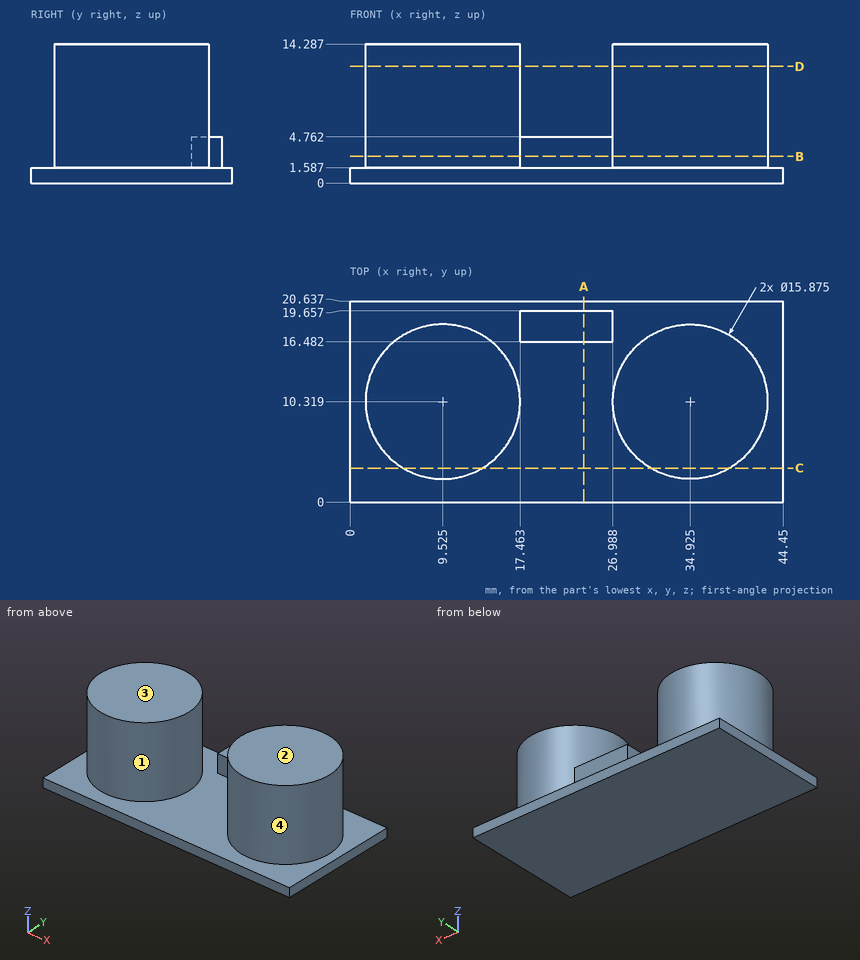
Could you check a few things on this drawing? It's one solid part, dimensions in mm from its lowest x, y, z. A direction names the side the tool comes from. Give positions to 0.01 mm unless a question says otherwise; leave off trailing zeros. Order: outer loops, then holes, each group sorted by start corner. A loop starts at its lowest first (then second) coordinate and runs counter-clockwise, first axis right, second up. Notation, with made-up numbers: (-12.75, 47) - (39.25, 47) arc R21 cw to (39.25, 71) - close; hole circle Ø8 at (6, 11). An arc over 180 degrees is marked (long way). Return JSON: item names as keys, results as strings. Group by question number.
Q1. Will these pins go through, and if not, where does the flat tip stop? pin 1 Ø3 at (y, z) = (18.5, 5) entering from -X; pin 2 Ø2.5 at (x, y) = (20, 17.5) entering from +Z; pin 3 Ø4 at (x, z) = (10.5, 6.5) entering from +Y.
Q2. Suppose I cut it at A-A, the plane x = 24. Please give me the cut outline in (y, z).
Q3. Which directions (+Z, -Z, +X, -X, +Y, -Y) give clear straight access to the entire face, cutting with the end or side of a thin tool? Please do the marked faces 1 and 2.
Q4. Suppose I cut it at B-B, the plane z = 2.75. Please give me the cut outline in (x, y) (1 decimal), and give its area (3 significant figures).
Q5. Please list where these lines run through material, in increasing order: line 1 along Z through (x, y) = (19.5, 1.5); line 2 along X through (y, z) = (6, 3.25) (1 decimal); line 3 along X through (y, z) = (5, 7.25) (1 decimal). Write a range as [from, to].
Q6. Thinking about a two-plate mould opening in X: for the marked faces 3 and 4, which applies, pulls with the +X half, pulls with the -X half, needs draft (parallel to the pull), parting line crosses it, or undercut?
Q7. Suppose I cut it at C-C, the plane y = 3.5. Please give me the cut outline in (x, z), and give its area (3 significant figures).
Q8. Suppose I cut it at D-D, the plane z = 12. Please give me the cut outline in (x, y) (1 decimal).
Resolved:
{
 "1": {"pin 1": "stops at x = 5.24", "pin 2": "stops at z = 4.76", "pin 3": "stops at y = 18.26"},
 "2": {"outline": "(0, 0) - (20.64, 0) - (20.64, 1.59) - (19.66, 1.59) - (19.66, 4.76) - (16.48, 4.76) - (16.48, 1.59) - (0, 1.59) - close"},
 "3": {"face 1": "+Z", "face 2": "+Z, +X, -X, +Y, -Y"},
 "4": {"outline": "circle Ø15.9 at (9.5, 10.3); (17.5, 16.5) - (27, 16.5) - (27, 19.7) - (17.5, 19.7) - close; circle Ø15.9 at (34.9, 10.3)", "area": "426 mm2"},
 "5": {"line 1": "z = [0, 1.59]", "line 2": "x = [2.9, 16.2], [28.3, 41.6]", "line 3": "x = [3.6, 15.4], [29, 40.8]"},
 "6": {"face 3": "needs draft", "face 4": "undercut"},
 "7": {"outline": "(0, 0) - (44.45, 0) - (44.45, 1.59) - (38.99, 1.59) - (38.99, 14.29) - (30.86, 14.29) - (30.86, 1.59) - (13.59, 1.59) - (13.59, 14.29) - (5.46, 14.29) - (5.46, 1.59) - (0, 1.59) - close", "area": "277 mm2"},
 "8": {"outline": "circle Ø15.9 at (9.5, 10.3); circle Ø15.9 at (34.9, 10.3)"}
}
